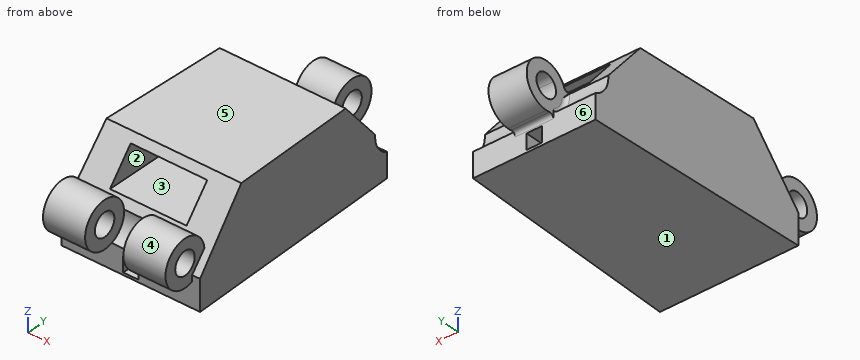
from build123d import *

# Parameters (mm, degrees)
BOSS_EXTRUDE2_DEPTH            = 12
CUT_EXTRUDE2_DEPTH             = 22.571014648
CUT_EXTRUDE2_DEPTH_BACK        = 22.571014648
BOSS_EXTRUDE3_DEPTH            = 2.5
CUT_EXTRUDE3_DEPTH             = 25.679395228
CUT_EXTRUDE3_DEPTH_BACK        = 25.679395228
SKETCH19_R                     = 3
SKETCH19_R_2                   = 1.5
BOSS_EXTRUDE4_DEPTH            = 8
SKETCH19_3_R                   = 3
CUT_EXTRUDE4_DEPTH             = 2.5
CUT_EXTRUDE5_START             = 10
SKETCH20_R                     = 3
CUT_EXTRUDE5_DEPTH             = 10
SKETCH21_R                     = 3
CUT_EXTRUDE6_DEPTH             = 10
FILLET6_R                      = 0.5
FILLET7_R                      = 0.5
FILLET8_R                      = 0.5
CUT_EXTRUDE7_REACH             = 27.076
SKETCH24_W                     = 10
SKETCH24_H                     = 3.849855631
CUT_EXTRUDE7_DIRECTION_2_REACH = 27.076
CUT_EXTRUDE8_DEPTH             = 1


with BuildPart() as part:
    # Sketch1 → Boss-Extrude2 (new body)
    with BuildSketch(Plane.XY):
        Polygon((-8, -14.5), (-6.966131725, 15.482179981), (9.033868275, 15.482179981), (10.06773655, -14.5), align=None)
    extrude(amount=BOSS_EXTRUDE2_DEPTH)

    # Sketch16 → Cut-Extrude2 (cut, two sides: drawn at the far end of the back side and taken through both)
    with BuildSketch(Plane(origin=(1.033868275, 0, 0), x_dir=(0, 0, -1), z_dir=(1, 0, 0)).offset(-CUT_EXTRUDE2_DEPTH_BACK)):
        Polygon((-12, 15.482179981), (-4, 15.482179981), (-12, 8.852541981), align=None)
    extrude(amount=CUT_EXTRUDE2_DEPTH + CUT_EXTRUDE2_DEPTH_BACK, mode=Mode.SUBTRACT)

    # Sketch17 → Boss-Extrude3 (add, symmetric)
    with BuildSketch(Plane(origin=(1.033868275, 0, 0), x_dir=(0, 0, -1), z_dir=(1, 0, 0))):
        with BuildLine():
            ThreePointArc((-8.791057147, 15.482179981), (-6, 13.582179981), (-3.208942853, 15.482179981))
            Line((-3.208942853, 15.482179981), (-4.980196097, 15.482179981))
            ThreePointArc((-4.980196097, 15.482179981), (-6, 15.082179981), (-7.019803903, 15.482179981))
            Line((-7.019803903, 15.482179981), (-8.791057147, 15.482179981))
        make_face()
        with BuildLine():
            Line((-4.980196097, 15.482179981), (-3.208942853, 15.482179981))
            ThreePointArc((-3.208942853, 15.482179981), (-3.05269857, 16.022345828), (-3, 16.582179981))
            ThreePointArc((-3, 16.582179981), (-6.559834153, 19.529481411), (-8.791057147, 15.482179981))
            Line((-8.791057147, 15.482179981), (-7.019803903, 15.482179981))
            ThreePointArc((-7.019803903, 15.482179981), (-6.600122548, 17.956899198), (-4.5, 16.582179981))
            ThreePointArc((-4.5, 16.582179981), (-4.625280782, 15.982057432), (-4.980196097, 15.482179981))
        make_face()
    extrude(amount=BOSS_EXTRUDE3_DEPTH, both=True)

    # Sketch18 → Cut-Extrude3 (cut, two sides: drawn at the far end of the back side and taken through both)
    with BuildSketch(Plane(origin=(1.033868275, 0, 0), x_dir=(0, 0, -1), z_dir=(1, 0, 0)).offset(-CUT_EXTRUDE3_DEPTH_BACK)):
        Polygon((-12, -7.870362001), (-12, -14.5), (-4, -14.5), align=None)
    extrude(amount=CUT_EXTRUDE3_DEPTH + CUT_EXTRUDE3_DEPTH_BACK, mode=Mode.SUBTRACT)

    # Sketch19 → Boss-Extrude4 (add, symmetric)
    with BuildSketch(Plane(origin=(1.033868275, 0, 0), x_dir=(0, 0, -1), z_dir=(1, 0, 0))):
        with Locations((-6, -15.6)):
            Circle(SKETCH19_R)
        with Locations((-6, -15.6)):
            Circle(SKETCH19_R_2, mode=Mode.SUBTRACT)
    extrude(amount=BOSS_EXTRUDE4_DEPTH, both=True)

    # Sketch19_3 → Cut-Extrude4 (cut, symmetric)
    with BuildSketch(Plane(origin=(1.033868275, 0, 0), x_dir=(0, 0, -1), z_dir=(1, 0, 0))):
        with Locations((-6, -15.6)):
            Circle(SKETCH19_3_R)
    extrude(amount=CUT_EXTRUDE4_DEPTH, both=True, mode=Mode.SUBTRACT)

    # Sketch20 → Cut-Extrude5 (cut)
    with BuildSketch(Plane(origin=(3.533868275, 0, 0), x_dir=(0, 0, -1), z_dir=(1, 0, 0)).offset(CUT_EXTRUDE5_START)):
        with Locations((-6, 16.582179981)):
            Circle(SKETCH20_R)
    extrude(amount=-CUT_EXTRUDE5_DEPTH, mode=Mode.SUBTRACT)

    # Sketch21 → Cut-Extrude6 (cut)
    with BuildSketch(Plane.ZY.offset(1.466131725)):
        with Locations((6, 16.582179981)):
            Circle(SKETCH21_R)
    extrude(amount=CUT_EXTRUDE6_DEPTH, mode=Mode.SUBTRACT)

    # Fillet6
    fillet6_edges = [part.edges().sort_by_distance(p)[0] for p in [
        (1.033868275, 13.595018046, 6.277242812),
    ]]
    fillet(fillet6_edges, radius=FILLET6_R)

    # Fillet7
    fillet7_edges = [part.edges().sort_by_distance(p)[0] for p in [
        (1.033868275, 15.482179981, 3.208942853),
    ]]
    fillet(fillet7_edges, radius=FILLET7_R)

    # Fillet8
    fillet8_edges = [part.edges().sort_by_distance(p)[0] for p in [
        (3.533868275, 14.026824951, 4.42832552),
        (-1.466131725, 14.026824951, 4.42832552),
    ]]
    fillet(fillet8_edges, radius=FILLET8_R)

    # Cut-Extrude7: up to this plane
    cut_extrude7_end = Plane(origin=(-8, -10.561614049, 8.752459729), z_dir=(0, 0.769971126082772, -0.6380787294674758))
    # Sketch24 → Cut-Extrude7 (cut, up to the surface)
    with BuildSketch(Plane(origin=(0, 0, 0), x_dir=(1, 0, 0), z_dir=(0, 1, 0)), mode=Mode.PRIVATE) as cut_extrude7_sk1:
        with Locations((1.033868275, -9.151106834)):
            Rectangle(SKETCH24_W, SKETCH24_H)
    cut_extrude7_tool1 = split(extrude(cut_extrude7_sk1.sketch, amount=-CUT_EXTRUDE7_REACH, mode=Mode.PRIVATE), bisect_by=cut_extrude7_end, keep=Keep.BOTH, mode=Mode.PRIVATE)
    add(cut_extrude7_tool1.solids().sort_by_distance((1.033868, 0, 9.151107))[0], mode=Mode.SUBTRACT)

    # Cut-Extrude7 direction 2: up to this plane
    cut_extrude7_direction_2_end = Plane(origin=(-8, 11.143904887, 9.235006912), z_dir=(0, 0.769971126082772, 0.6380787294674758))
    # Sketch24 → Cut-Extrude7 direction 2 (cut, up to the surface)
    with BuildSketch(Plane(origin=(0, 0, 0), x_dir=(1, 0, 0), z_dir=(0, 1, 0)), mode=Mode.PRIVATE) as cut_extrude7_direction_2_sk1:
        with Locations((1.033868275, -9.151106834)):
            Rectangle(SKETCH24_W, SKETCH24_H)
    cut_extrude7_direction_2_tool1 = split(extrude(cut_extrude7_direction_2_sk1.sketch, amount=CUT_EXTRUDE7_DIRECTION_2_REACH, mode=Mode.PRIVATE), bisect_by=cut_extrude7_direction_2_end, keep=Keep.BOTH, mode=Mode.PRIVATE)
    add(cut_extrude7_direction_2_tool1.solids().sort_by_distance((1.033868, 0, 9.151107))[0], mode=Mode.SUBTRACT)

    # Sketch25 → Cut-Extrude8 (cut, symmetric)
    with BuildSketch(Plane(origin=(1.033868275, 0, 0), x_dir=(0, 0, -1), z_dir=(1, 0, 0))):
        Polygon((-2.32, -14.5), (-0.32, -14.5), (-0.32, -14.381743642), (-0.32, 15.88316041), (-2.32, 15.88316041), (-2.32, -14.381743642), align=None)
    extrude(amount=CUT_EXTRUDE8_DEPTH, both=True, mode=Mode.SUBTRACT)


solid = part.part
Geometry: final body of the model. Coordinates: model frame, mm. Face numbers are marked on the shaded views. A direction names the side the tool comes from. Give positions to 0.01 mm unless a question says otherwise; leave off trailing zeros. Write each loop counter-clockwise with the first axis right and the second up, starting at its lowest first coordinate (ties: lowest second). Pieces come first, ordered by that corner, then holes. Notation, with made-up numbers: (-31.75, 26.25) -> (4.25, 26.25) arc R27 cw to (4.25, 61.25) -> close; hole circle Ø3 at (5.5, -2.5). An arc over 180 degrees is marked (long way). Answer in a Markdown table with one row per item.
(1) Section query D-D on x = 0.5. Return loops of the section in (y, z) (3 decimals).
Answers below:
| item | result |
|---|---|
| outline | (-14.5, 0) -> (15.482, 0) -> (15.482, 0.32) -> (-14.5, 0.32) -> close; (-14.5, 2.32) -> (15.482, 2.32) -> (15.482, 2.552) arc R0.5 cw to (16.068, 3.044) arc R3 ccw (long way) to (13.815, 7.159) arc R0.5 cw to (12.969, 7.033) -> (12.809, 7.226) -> (-11.826, 7.226) -> (-12.613, 6.277) arc R3 cw to (-14.5, 3.209) -> close; (-8.636, 11.076) -> (9.618, 11.076) -> (8.853, 12) -> (-7.87, 12) -> close; hole circle Ø3 at (16.582, 6) |
(2) Ray query, line 1 along Z through (x, y) = (6, 2); line 2 along Y through (x, z) = (1.8, 6); line 3 along Y through (x, z) = (7.4, 6). Return the intervals inside material, ascending. Write a range as [from, to].
Answers below:
| item | result |
|---|---|
| line 1 | [0, 7.23], [11.08, 12] |
| line 2 | [-12.6, 15.08], [18.08, 19.58] |
| line 3 | [-18.6, -17.1], [-14.1, 13.58] |
(3) Section query B-B on x = -2.75. Return loops of the section in (y, z), then the cut area to 3 significant figures.
Answers below:
| item | result |
|---|---|
| outline | (-14.5, 0) -> (15.48, 0) -> (15.48, 3.21) arc R3 cw to (13.6, 6.28) -> (12.81, 7.23) -> (-11.83, 7.23) -> (-12.61, 6.28) arc R3 ccw (long way) to (-14.5, 3.21) -> close; (-8.64, 11.08) -> (9.62, 11.08) -> (8.85, 12) -> (-7.87, 12) -> close; hole circle Ø3 at (-15.6, 6) |
| area | 241 mm^2 |
(4) Section query C-C on z = 1. Return loops of the section in (x, y), then the cut area to 3 significant figures.
Answers below:
| item | result |
|---|---|
| outline | (-8, -14.5) -> (0.03, -14.5) -> (0.03, 15.48) -> (-6.97, 15.48) -> close; (2.03, -14.5) -> (10.07, -14.5) -> (9.03, 15.48) -> (2.03, 15.48) -> close |
| area | 451 mm^2 |
(5) Draft query along Y for the marked faces 4, 5 and 6. Return one class per face: +Y half, -Y half, draft (parallel to the pull), parting line (faces both ways), or undercut.
Answers below:
| item | result |
|---|---|
| face 4 | undercut |
| face 5 | draft |
| face 6 | +Y half |
(6) Section query A-A on y = -15.6. Return loops of the section in (x, z), then the cut area to 3 significant figures.
Answers below:
| item | result |
|---|---|
| outline | (-6.97, 3) -> (-1.47, 3) -> (-1.47, 4.5) -> (-6.97, 4.5) -> close; (-6.97, 7.5) -> (-1.47, 7.5) -> (-1.47, 9) -> (-6.97, 9) -> close; (3.53, 3) -> (9.03, 3) -> (9.03, 4.5) -> (3.53, 4.5) -> close; (3.53, 7.5) -> (9.03, 7.5) -> (9.03, 9) -> (3.53, 9) -> close |
| area | 33.0 mm^2 |
(7) Pin query (flat end, axial travel): pin 1 (6 mm diameter, centred on y = 7.5, z = 5, fed in from +X); pin 2 (3 mm diameter, centred on y = 6.5, z = 8, fed in from -X); pin 3 (1.5 mm diameter, centred on x = 0.5, z = 1.5, fed in from +Y); pin 4 (2.5 mm diameter, centred on y = -15.6, z = 6, fed in from +X). Return the tip coordinate at first contact, or that it passes through.
Answers below:
| item | result |
|---|---|
| pin 1 | x = 9.41 |
| pin 2 | x = -7.33 |
| pin 3 | y = 15.48 |
| pin 4 | through |
(8) Set-up query: the marked faces 1, 2 and 3. Return all of +Z, -Z, +X, -X, +Y, -Y with unobstructed straight access to the full face (end or side cutting, diameter ignored); none if empty.
Answers below:
| item | result |
|---|---|
| face 1 | -Z, +X, -X, +Y, -Y |
| face 2 | +Y |
| face 3 | none |
